from build123d import *

# Parameters (mm, degrees)
SKETCH004_R  = 6
PAD003_DEPTH = 60
SKETCH005_R  = 1.5
PAD004_DEPTH = 10
SKETCH003_R  = 7.46
PAD002_DEPTH = 25
SKETCH_W     = 60
SKETCH_H     = 105
SKETCH_W_2   = 43
SKETCH_H_2   = 64
PAD_DEPTH    = 5
PAD001_DEPTH = 5
CHAMFER_SIZE = 15


with BuildPart() as rodmount:
    # Sketch004 → Pad003 (new body)
    with BuildSketch(Plane.YZ):
        with Locations((10, 10)):
            Circle(SKETCH004_R)
        with Locations((95, 10)):
            Circle(SKETCH004_R)
    extrude(amount=PAD003_DEPTH)


with BuildPart() as basemountpoints:
    # Sketch005 → Pad004 (new body)
    with BuildSketch(Plane.XY.offset(10)):
        with Locations((4, 19.25)):
            Circle(SKETCH005_R)
        with Locations((56, 19.25)):
            Circle(SKETCH005_R)
        with Locations((56, 85.75)):
            Circle(SKETCH005_R)
        with Locations((4, 85.75)):
            Circle(SKETCH005_R)
    extrude(amount=-PAD004_DEPTH)


with BuildPart() as cutblocks:
    # Sketch003 → Pad002 (new body)
    with BuildSketch(Plane.YZ.offset(17.5)):
        with Locations((10, 10)):
            Circle(SKETCH003_R)
        with Locations((95, 10)):
            Circle(SKETCH003_R)
    extrude(amount=PAD002_DEPTH)

    # Fusion: union RodMount, BaseMountPoints
    add(rodmount.part)
    add(basemountpoints.part)


with BuildPart() as base:
    # Sketch → Pad (new body)
    with BuildSketch(Plane.XY):
        with Locations((30, 52.5)):
            Rectangle(SKETCH_W, SKETCH_H)
        with Locations((30, 50.5)):
            Rectangle(SKETCH_W_2, SKETCH_H_2, mode=Mode.SUBTRACT)
    extrude(amount=PAD_DEPTH)


with BuildPart() as chamfer_body:
    # Pad001 base: copy of Base
    add(base.part)

    # Sketch001 → Pad001 (new body)
    with BuildSketch(Plane.XY.offset(5)):
        Polygon((16.5, 105), (43.5, 105), (43.5, 92.5), (60, 92.5), (60, 82.5), (0, 82.5), (0, 92.5), (16.5, 92.5), align=None)
        Polygon((43.5, 0), (16.5, 0), (16.5, 12.5), (0, 12.5), (0, 22.5), (8.5, 22.5), (8.5, 18.5), (51.5, 18.5), (51.5, 22.5), (60, 22.5), (60, 12.5), (43.5, 12.5), align=None)
    extrude(amount=PAD001_DEPTH)

    # Fusion001: union Base
    add(base.part)

    # Cut: cut CutBlocks
    add(cutblocks.part, mode=Mode.SUBTRACT)

    # Chamfer
    chamfer_edges = [chamfer_body.edges().sort_by_distance(p)[0] for p in [
        (60, 105, 2.5),
        (0, 105, 2.5),
        (60, 0, 2.5),
        (0, 0, 2.5),
    ]]
    chamfer(chamfer_edges, length=CHAMFER_SIZE)


solid = chamfer_body.part
Geometry check sheet. Reference: the model listing, model coordinates, mm. A direction names the side the tool comes from. Give positions to 0.01 mm unless a question says otherwise; leave off trailing zeros. Loops run counter-clockwise (first coordinate to the right, second up) from the corner with the lowest first, then second, coordinate; pieces in that order, holes last. Notation, with made-up numbers: M 50,-38 L 86,-38 A23 cw 86,-25 Z; hole C 0,56 d10. An arc over 180 degrees is marked long. Answer as a JSON object with one key per item and string values. Group by question number.
Item 1: Mould release check, pull along X, two halves, no side actions. Record for faces 6 (the flat face through (8, 7, 3)), 7 (the flat face through (30, 86, 10)), 8 (the flat face through (42.5, 9.4, 3.8)): pulls with the +X half, pulls with the -X half, needs draft (parallel to the pull), parting line crosses it, or undercut.
Item 2: Access from +Z, -Z, +X, -X, +Y, -Y to the whole of each face (thin tool, end or side, straight path). Record for faces 1 (the flat face through (43.5, 3, 7)), 2 (the flat face through (4, 53, 5)), 3 (the flat face through (51.5, 50, 3)), 4 (the flat face through (43.5, 102, 7)), 5 (the flat face through (16.5, 102, 7)).
Item 3: Gauge pin test, flat ends, axial feed: pin 1 (5.5 mm diameter, centred on x = 48, y = 102, fed in from +Z); pin 2 (2 mm diameter, centred on x = 6.5, z = 4.5, fed in from +Y); pin 3 (2.5 mm diameter, centred on x = 2.5, z = 7, fed in from +Y). Record the tip position at first contact, or that the pin passes through.
Item 4: Material ranges on L1, parallel to X at y = 85.75, z = 6.5; L2, parallel to Y at x = 56, z = 6.75; L3, parallel to X at y = 25.5, z = 4, recorded low to high.
Item 5: Sectioned sample at D-D on x = 4. Record the boundary of the cut face in (y, z), plus the area to 3 significant figures.
Item 6: Sectioned sample at C-C on y = 38. Record the boundary of the cut face in (x, z).
Item 7: Sectioned sample at B-B on z = 1. Record the boundary of the cut face in (x, y), plus the area to 3 significant figures.
Item 8: Sectioned sample at A-A on x = 31. Record the boundary of the cut face in (y, z).
Findings below:
{
 "1": {"face 6": "pulls with the -X half", "face 7": "needs draft", "face 8": "undercut"},
 "2": {"face 1": "+Z, +X, -Y", "face 2": "+Z, +X, -X", "face 3": "+Z, -Z", "face 4": "+Z, +X, +Y", "face 5": "+Z, -X, +Y"},
 "3": {"pin 1": "z = 5", "pin 2": "y = 97.5", "pin 3": "y = 90.76"},
 "4": {"L1": "0 to 2.5, 5.5 to 54.5, 57.5 to 60", "L2": "15.04 to 17.75, 20.75 to 22.5, 82.5 to 84.25, 87.25 to 89.96", "L3": "0 to 8.5, 51.5 to 60"},
 "5": {"outline": "M 11,0 L 17.75,0 L 17.75,10 L 16,10 A6 cw 11,4.08 Z; M 20.75,0 L 84.25,0 L 84.25,10 L 82.5,10 L 82.5,5 L 22.5,5 L 22.5,10 L 20.75,10 Z; M 87.25,0 L 94,0 L 94,4.08 A6 cw 89,10 L 87.25,10 Z", "area": "425 mm2"},
 "6": {"outline": "M 0,0 L 8.5,0 L 8.5,5 L 0,5 Z; M 51.5,0 L 60,0 L 60,5 L 51.5,5 Z"},
 "7": {"outline": "M 0,15 L 15,0 L 45,0 L 60,15 L 60,90 L 45,105 L 15,105 L 0,90 Z; hole C 4,19.25 d3; hole C 4,85.75 d3; hole M 8.5,18.5 L 51.5,18.5 L 51.5,82.5 L 8.5,82.5 Z; hole C 56,19.25 d3; hole C 56,85.75 d3", "area": "3,070 mm2"},
 "8": {"outline": "M 0,0 L 18.5,0 L 18.5,10 L 17.46,10 A7.46 cw 2.54,10 L 0,10 Z; M 82.5,0 L 105,0 L 105,10 L 102.46,10 A7.46 cw 87.54,10 L 82.5,10 Z"}
}
